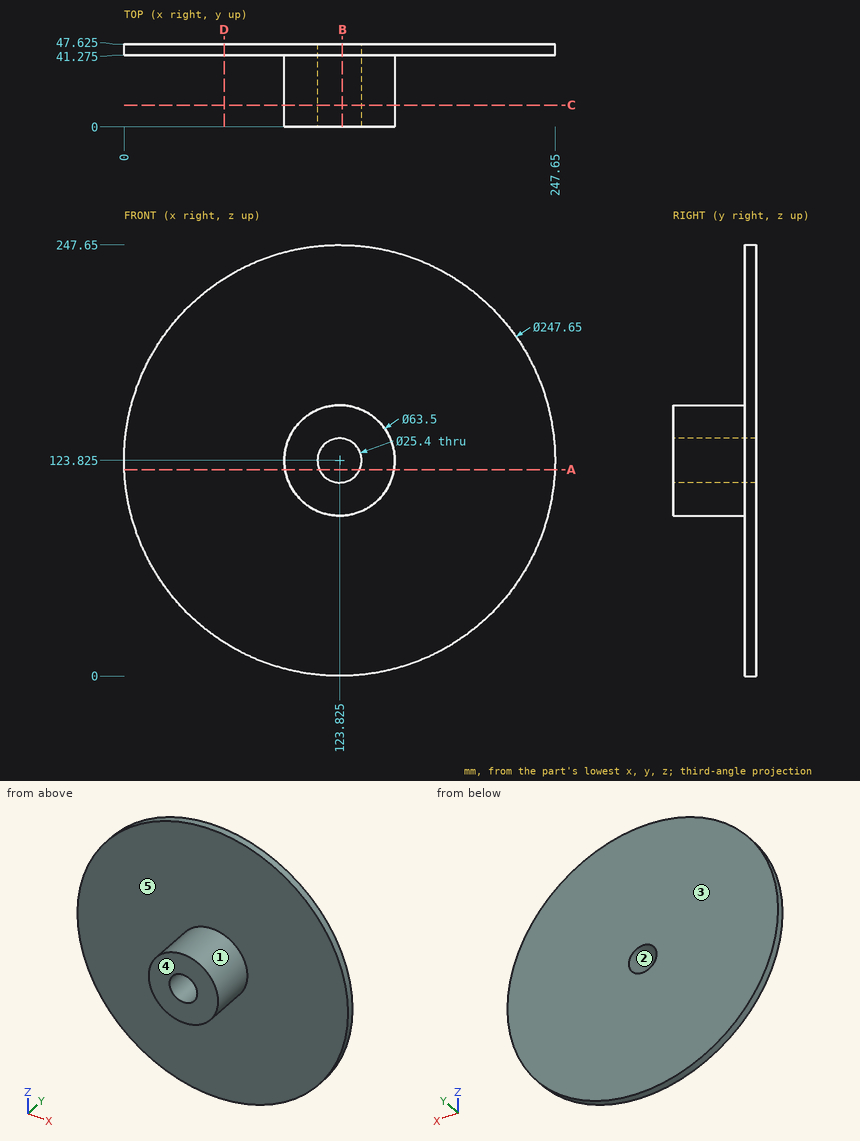
Job drawing, mm, ordinate dimensions from the low corner. One solid piece. A direction names the side the tool comes from. Give positions to 0.01 mm unless a question says otherwise; leave off trailing zeros. Loops run counter-clockwise (first coordinate to the right, second up) from the corner with the lowest first, then second, coordinate; pieces in that order, holes last. Notation, with made-up numbers: (24.25, 44) -> (67.25, 44) arc R32 ccw to (67.25, 83) -> close; hole circle Ø5 at (58, 67). An arc over 180 degrees is marked (long way). Use a Markdown table: item, result. Add a question column.
(1) Slice it at B-B on x = 125.5. List the corners of the cut face in (y, z) (3 decimals).
(2) Slice it at C-C on y = 12.5. List the corners of the cut face in (x, z) (3 decimals).
(3) Tool access for the marked faces 4 and 5: list every direction of +Z, -Z, +X, -X, +Y, -Y with a clear straight run to the whole face (end or side of a thin tool).
(4) Mould opens along Z. For the marked faces 1, 2 and 3 say: +Z half, -Z half, draft (parallel to the pull), parting line (faces both ways), or undercut.
(5) Slice it at D-D on x = 57.5. List the corners of the cut face in (y, z) (3 decimals), and give its area (3 significant figures).
(6) Wall check: line 1 along Y through (x, z) = (76.5, 121) (3 decimals); line 2 along X through (y, z) = (13, 134.5) (3 decimals); line 3 along Z through (x, y) = (117, 35). Give the ranges that are in metal, low to high.
(7) Slice it at A-A on z = 118.5. List the corners of the cut face in (x, y) (3 decimals).
(8) Drop flat-ended pins along their axis: pin 1 Ø5 at (y, z) = (22, 143) entering from +X; pin 2 Ø2 at (x, z) = (149.5, 29.5) entering from -Y (3 decimals). Give the stop position or say it passes through.
Filled sheet:
| question | item | result |
|---|---|---|
| 1 | outline | (0, 92.119) -> (41.275, 92.119) -> (41.275, 0.011) -> (47.625, 0.011) -> (47.625, 111.236) -> (0, 111.236) -> close; (0, 136.414) -> (47.625, 136.414) -> (47.625, 247.639) -> (41.275, 247.639) -> (41.275, 155.531) -> (0, 155.531) -> close |
| 2 | outline | circle Ø63.5 at (123.825, 123.825); hole circle Ø25.4 at (123.825, 123.825) |
| 3 | face 4 | +Z, -Z, +X, -X, -Y |
| 3 | face 5 | -Y |
| 4 | face 1 | parting line |
| 4 | face 2 | undercut |
| 4 | face 3 | draft |
| 5 | outline | (41.275, 19.261) -> (47.625, 19.261) -> (47.625, 228.389) -> (41.275, 228.389) -> close |
| 5 | area | 1,330 mm2 |
| 6 | line 1 | 41.275 to 47.625 |
| 6 | line 2 | 93.923 to 116.945, 130.705 to 153.727 |
| 6 | line 3 | 92.82 to 113.11, 134.54 to 154.83 |
| 7 | outline | (0.115, 41.275) -> (92.525, 41.275) -> (92.525, 0) -> (112.295, 0) -> (112.295, 47.625) -> (0.115, 47.625) -> close; (135.355, 0) -> (155.125, 0) -> (155.125, 41.275) -> (247.535, 41.275) -> (247.535, 47.625) -> (135.355, 47.625) -> close |
| 8 | pin 1 | x = 150.84 |
| 8 | pin 2 | y = 41.275 |
